Read the model definition and answer for the solid it produces. Units are mm, in the model's axes. Coordinates: 2 decimals unless noted, no trailing zeros. Write each loop counter-clockwise with the first axis right and the second up, starting at its lowest first coordinate (ties: lowest second). Pieces come first, ordered by that corner, then holes. Notation, with made-up numbers: (-23, 54.5) - (-10, 54.5) arc R19 ccw to (-10, 87.5) - close; hole circle Ø7 at (75.5, 37). An arc over 180 degrees is marked (long way). Return JSON: item names as keys, results as strings.
```python
from build123d import *

# Parameters (mm, degrees)
F0_W          = 50
F0_H          = 50
F0_W_2        = 40
F0_H_2        = 40
F1_DEPTH      = 3000
F3_DEPTH      = 25.001
F3_DEPTH_BACK = 25.001
F4_R          = 7.5
F5_DEPTH      = 50.001


with BuildPart() as f1:
    # F0 (on Front) → F1 (new body)
    with BuildSketch(Plane.XZ):
        Rectangle(F0_W, F0_H)
        Rectangle(F0_W_2, F0_H_2, mode=Mode.SUBTRACT)
    extrude(amount=-F1_DEPTH)

    # F2 (on Top) → F3 (cut, two sides)
    with BuildSketch(Plane.XY) as f3_sk:
        Polygon((-25, 3000), (-25, 2849.7744184879), (25, 2736.739757117), (25, 3000), align=None)
        Polygon((25, 22.1171096519), (-25, 0), (25, 0), align=None)
    extrude(amount=-F3_DEPTH, mode=Mode.SUBTRACT)
    extrude(f3_sk.sketch, amount=F3_DEPTH_BACK, mode=Mode.SUBTRACT)

    # F4 (on face) → F5 (cut, through all)
    with BuildSketch(Plane.XY.offset(25)):
        with Locations((-7.9764017243, 34.8668911918)):
            Circle(F4_R)
    extrude(amount=-F5_DEPTH, mode=Mode.SUBTRACT)


solid = f1.part
```
(1) Flat-ended cylindrical pins translate along their axes: P1, Ø8, axis at x = -3.5, z = 20, coming from the +Y side; P2, Ø13.5, axis at x = -7.98, y = 34.87, coming from the +Z side. Find the tip coordinate at first contact, or state that the pin passes through.
Answer:
{"P1": "y = 2810.21", "P2": "through"}
(2) Straight lines are drawn through the part: line 1 (Z direction, x = -14, y = 1487); line 2 (Y direction, x = -23, z = 17). For each, find the intervals that lie inside material, in ascending order. Write a range as from..to.
Answer:
{"line 1": "-25..-20, 20..25", "line 2": "0.88..2845.25"}
(3) A cutting plane is placed at B-B (y = 1605.5). Determine the outline of the cut face in (x, z), and give its area (3 significant figures).
Answer:
{"outline": "(-25, -25) - (25, -25) - (25, 25) - (-25, 25) - close; hole (-20, -20) - (20, -20) - (20, 20) - (-20, 20) - close", "area": "900 mm²"}
(4) A cutting plane is placed at C-C (x = 8). Determine the outline of the cut face in (y, z), and give its area (3 significant figures).
Answer:
{"outline": "(14.6, -25) - (2775.17, -25) - (2775.17, -20) - (14.6, -20) - close; (14.6, 20) - (2775.17, 20) - (2775.17, 25) - (14.6, 25) - close", "area": "27,600 mm²"}
(5) A cutting plane is placed at A-A (z = 5). Determine the outline of the cut face in (x, y).
Answer:
{"outline": "(-25, 0) - (-20, 2.21) - (-20, 2838.47) - (-25, 2849.77) - close; (20, 19.91) - (25, 22.12) - (25, 2736.74) - (20, 2748.04) - close"}
